from build123d import *

# Parameters (mm, degrees)
SKETCH_1_R               = 38.15
EXTRUDE_1_DEPTH          = 3
SKETCH_2_R               = 35.35
EXTRUDE_2_DEPTH          = 2
SKETCH_6_R               = 5.5
CUT_EXTRUDE_2_DEPTH      = 6
SKETCH_7_R               = 32.5
SKETCH_7_R_2             = 13.5
CUT_EXTRUDE_3_DEPTH      = 1
CUT_EXTRUDE_3_DEPTH_BACK = 6
EXTRUDE_4_DEPTH          = 5
PATTERN_CIRCULAR_3_COUNT = 6
MIRROR_1_COPY_1_DEPTH    = 5
MIRROR_1_COPY_2_DEPTH    = 5
MIRROR_1_COPY_3_DEPTH    = 5
MIRROR_1_COPY_4_DEPTH    = 5
MIRROR_1_COPY_5_DEPTH    = 5
SKETCH_9_R               = 1.6
CUT_EXTRUDE_4_DEPTH      = 6
FILLET_3_R               = 1.6
FILLET_4_R               = 1.6
SKETCH_11_R              = 12.05
CUT_EXTRUDE_6_DEPTH      = 2


with BuildPart() as part:
    # ｽｹｯﾁ1 → ﾎﾞｽ - 押し出し1 (new body)
    with BuildSketch(Plane.XY):
        Circle(SKETCH_1_R)
    extrude(amount=EXTRUDE_1_DEPTH)

    # ｽｹｯﾁ2 → ﾎﾞｽ - 押し出し2 (add)
    with BuildSketch(Plane.XY.offset(3)):
        Circle(SKETCH_2_R)
    extrude(amount=EXTRUDE_2_DEPTH)

    # ｽｹｯﾁ6 → ｶｯﾄ - 押し出し2 (cut, through all)
    with BuildSketch(Plane.XY.offset(5)):
        Circle(SKETCH_6_R)
    extrude(amount=-CUT_EXTRUDE_2_DEPTH, mode=Mode.SUBTRACT)

    # ｽｹｯﾁ7 → ｶｯﾄ - 押し出し3 (cut, two sides)
    with BuildSketch(Plane.XY.offset(5)) as cut_extrude_3_sk:
        Circle(SKETCH_7_R)
        Circle(SKETCH_7_R_2, mode=Mode.SUBTRACT)
    extrude(amount=CUT_EXTRUDE_3_DEPTH, mode=Mode.SUBTRACT)
    extrude(cut_extrude_3_sk.sketch, amount=-CUT_EXTRUDE_3_DEPTH_BACK, mode=Mode.SUBTRACT)

    # ｽｹｯﾁ8 → ﾎﾞｽ - 押し出し4 (add)
    with BuildSketch(Plane.XY.offset(5)):
        with BuildLine():
            Line((-12.910378376, 3.946153846), (-4.268742546, 32.218439395))
            ThreePointArc((-4.268742546, 32.218439395), (-2.139009075, 32.429533456), (0, 32.5))
            Line((0, 32.5), (-6.281364189, 11.949663758))
            ThreePointArc((-6.281364189, 11.949663758), (-10.396864354, 8.611342032), (-12.910378376, 3.946153846))
        make_face()
    extrude_4 = extrude(amount=-EXTRUDE_4_DEPTH)

    # 円形ﾊﾟﾀｰﾝ3: ﾎﾞｽ - 押し出し4 ×6 about axis
    pattern_circular_3_axis = Axis((0, 0, 0), (0, 0, 1))
    for i in range(1, PATTERN_CIRCULAR_3_COUNT):
        add(extrude_4.rotate(pattern_circular_3_axis, i * 360 / PATTERN_CIRCULAR_3_COUNT))

    # ﾐﾗｰ1: ﾎﾞｽ - 押し出し4 across plane
    add(extrude_4.mirror(Plane(origin=(0, 0, 0), x_dir=(0, 0, 1), z_dir=(1, 0, 0))))

    # ﾐﾗｰ1 copy 1 sketch → ﾐﾗｰ1 copy 1 (add)
    with BuildSketch(Plane(origin=(0, 0, 5), x_dir=(-0.5, 0.866025404, 0), z_dir=(0, 0, 1))):
        with BuildLine():
            Line((-12.910378376, -3.946153846), (-4.268742546, -32.218439395))
            ThreePointArc((-4.268742546, -32.218439395), (-2.139009075, -32.429533456), (0, -32.5))
            Line((0, -32.5), (-6.281364189, -11.949663758))
            ThreePointArc((-6.281364189, -11.949663758), (-10.396864354, -8.611342032), (-12.910378376, -3.946153846))
        make_face()
    extrude(amount=-MIRROR_1_COPY_1_DEPTH)

    # ﾐﾗｰ1 copy 2 sketch → ﾐﾗｰ1 copy 2 (add)
    with BuildSketch(Plane(origin=(0, 0, 5), x_dir=(0.5, 0.866025404, 0), z_dir=(0, 0, 1))):
        with BuildLine():
            Line((-12.910378376, -3.946153846), (-4.268742546, -32.218439395))
            ThreePointArc((-4.268742546, -32.218439395), (-2.139009075, -32.429533456), (0, -32.5))
            Line((0, -32.5), (-6.281364189, -11.949663758))
            ThreePointArc((-6.281364189, -11.949663758), (-10.396864354, -8.611342032), (-12.910378376, -3.946153846))
        make_face()
    extrude(amount=-MIRROR_1_COPY_2_DEPTH)

    # ﾐﾗｰ1 copy 3 sketch → ﾐﾗｰ1 copy 3 (add)
    with BuildSketch(Plane.XY.offset(5)):
        with BuildLine():
            Line((-12.910378376, -3.946153846), (-4.268742546, -32.218439395))
            ThreePointArc((-4.268742546, -32.218439395), (-2.139009075, -32.429533456), (0, -32.5))
            Line((0, -32.5), (-6.281364189, -11.949663758))
            ThreePointArc((-6.281364189, -11.949663758), (-10.396864354, -8.611342032), (-12.910378376, -3.946153846))
        make_face()
    extrude(amount=-MIRROR_1_COPY_3_DEPTH)

    # ﾐﾗｰ1 copy 4 sketch → ﾐﾗｰ1 copy 4 (add)
    with BuildSketch(Plane(origin=(0, 0, 5), x_dir=(0.5, -0.866025404, 0), z_dir=(0, 0, 1))):
        with BuildLine():
            Line((-12.910378376, -3.946153846), (-4.268742546, -32.218439395))
            ThreePointArc((-4.268742546, -32.218439395), (-2.139009075, -32.429533456), (0, -32.5))
            Line((0, -32.5), (-6.281364189, -11.949663758))
            ThreePointArc((-6.281364189, -11.949663758), (-10.396864354, -8.611342032), (-12.910378376, -3.946153846))
        make_face()
    extrude(amount=-MIRROR_1_COPY_4_DEPTH)

    # ﾐﾗｰ1 copy 5 sketch → ﾐﾗｰ1 copy 5 (add)
    with BuildSketch(Plane(origin=(0, 0, 5), x_dir=(-0.5, -0.866025404, 0), z_dir=(0, 0, 1))):
        with BuildLine():
            Line((-12.910378376, -3.946153846), (-4.268742546, -32.218439395))
            ThreePointArc((-4.268742546, -32.218439395), (-2.139009075, -32.429533456), (0, -32.5))
            Line((0, -32.5), (-6.281364189, -11.949663758))
            ThreePointArc((-6.281364189, -11.949663758), (-10.396864354, -8.611342032), (-12.910378376, -3.946153846))
        make_face()
    extrude(amount=-MIRROR_1_COPY_5_DEPTH)

    # ｽｹｯﾁ9 → ｶｯﾄ - 押し出し4 (cut, through all)
    with BuildSketch(Plane.XY.offset(5)):
        with Locations((-8.5, 0)):
            Circle(SKETCH_9_R)
        with Locations((0, 8.5)):
            Circle(SKETCH_9_R)
        with Locations((8.5, 0)):
            Circle(SKETCH_9_R)
        with Locations((0, -8.5)):
            Circle(SKETCH_9_R)
    extrude(amount=-CUT_EXTRUDE_4_DEPTH, mode=Mode.SUBTRACT)

    # ﾌｨﾚｯﾄ3
    fillet_3_edges = [part.edges().sort_by_distance(p)[0] for p in [
        (11.999058751, 6.9276598, 2.5),
        (9.230036516, 15.986892202, 2.5),
        (4.268742546, 32.218439395, 2.5),
        (15.725247398, -2.932347892, 2.5),
        (15.725247398, 2.932347892, 2.5),
        (18.460073032, 0, 2.5),
        (11.999058751, -6.9276598, 2.5),
        (30.03635826, 12.41238021, 2.5),
        (10.402111466, -12.152289781, 2.5),
        (9.230036516, -15.986892202, 2.5),
        (25.767615714, -19.806059185, 2.5),
        (-5.323135932, 15.084637673, 2.5),
        (-9.230036516, 15.986892202, 2.5),
        (0, 13.8553196, 2.5),
        (-25.767615714, 19.806059185, 2.5),
        (4.268742546, -32.218439395, 2.5),
        (30.03635826, -12.41238021, 2.5),
        (28.145825623, -16.25, 2.5),
        (25.767615714, 19.806059185, 2.5),
        (28.145825623, 16.25, 2.5),
        (-4.268742546, 32.218439395, 2.5),
        (0, 32.5, 2.5),
        (10.402111466, 12.152289781, 2.5),
        (5.323135932, 15.084637673, 2.5),
    ]]
    fillet(fillet_3_edges, radius=FILLET_3_R)

    # ﾌｨﾚｯﾄ4
    fillet_4_edges = [part.edges().sort_by_distance(p)[0] for p in [
        (5.323135932, -15.084637673, 2.5),
        (0, -13.8553196, 2.5),
        (-10.402111466, -12.152289781, 2.5),
        (-5.323135932, -15.084637673, 2.5),
        (-9.230036516, -15.986892202, 2.5),
        (-11.999058751, -6.9276598, 2.5),
        (-4.268742546, -32.218439395, 2.5),
        (-15.725247398, 2.932347892, 2.5),
        (-15.725247398, -2.932347892, 2.5),
        (-18.460073032, 0, 2.5),
        (-11.999058751, 6.9276598, 2.5),
        (-30.03635826, -12.41238021, 2.5),
        (-30.03635826, 12.41238021, 2.5),
        (-28.145825623, 16.25, 2.5),
        (-10.402111466, 12.152289781, 2.5),
        (-25.767615714, -19.806059185, 2.5),
        (-28.145825623, -16.25, 2.5),
        (0, -32.5, 2.5),
    ]]
    fillet(fillet_4_edges, radius=FILLET_4_R)

    # ｽｹｯﾁ11 → ｶｯﾄ - 押し出し6 (cut)
    with BuildSketch(Plane.XY.offset(5)):
        Circle(SKETCH_11_R)
    extrude(amount=-CUT_EXTRUDE_6_DEPTH, mode=Mode.SUBTRACT)


solid = part.part
The model under review builds one solid part; all positions refer to its coordinate system, in mm. A direction names the side the tool comes from. Round coordinates to 2 decimals unless told otherwise and drop trailing zeros. Write each loop counter-clockwise with the first axis right and the second up, starting at its lowest first coordinate (ties: lowest second). Pieces come first, ordered by that corner, then holes. Notation, with made-up numbers: M 22,-28.75 L 50,-28.75 A26 ccw 50,-4.75 Z; hole C 49.5,23 d3. An arc over 180 degrees is marked long. Use a Markdown table: item, result. Add a question column.
Q1. We need section B-B, the plane y = -25. State the section outline as (x, z) points, plus the area to 3 significant figures.
Q2. Machinability: for faces 1 (the face through (32.5, -0.1, 2.5)), 2 (the face through (-8.881, 8.144, 4.014)), which of the approach directions +Z, -Z, +X, -X, +Y, -Y give a long, thin tool a straight path to every point of the face, cutting with its end or side? Answer none if there is none.
Q3. The part is to be moulded in two halves that separate along Y. For faces 3 (the face through (24.39, -20.28, 2.46)), 4 (the face through (33.718, 10.618, 3.986)), 5 (the face through (15.74, -3.68, 2.46)), 6 (the face through (9, 14, 5)), say which applies: pulls with the +Y half, pulls with the -Y half, needs draft (parallel to the pull), parting line crosses it, or undercut.
Q4. Insertion check: pin 1 (1 mm diameter, centred on x = 10.5, z = 2, fed in from +Y); pin 2 (1 mm diameter, centred on y = -25, z = 4, fed in from +X); pin 3 (1 mm diameter, centred on x = -14.5, y = 16, fed in from -Z); pin 4 (3 mm diameter, centred on x = 8.5, y = 0, fed in from -Z). Each pin has a flat end and moves straight along its axis. Give the tip position at first contact, or say it passes through.
Q5. We need section A-A, the plane y = 0. Count the separate pieces of the cut face and the enclosed holes in it, plus the area to 3 significant figures.
Q6. To check wall thickness, follow line 1 (X direction, y = -29, z = 3.45); line 2 (X direction, y = 3.5, z = 1.3); line 3 (X direction, y = 24, z = 3.2). State the ranges of each line that lie inside material, in increasing order.
Findings below:
| question | item | result |
|---|---|---|
| 1 | outline | M -28.82,0 L -20.77,0 L -20.77,5 L -24.99,5 L -24.99,3 L -28.82,3 Z; M -6.48,0 L -2.29,0 L -2.29,5 L -6.48,5 Z; M 2.29,0 L 6.48,0 L 6.48,5 L 2.29,5 Z; M 20.77,0 L 28.82,0 L 28.82,3 L 24.99,3 L 24.99,5 L 20.77,5 Z |
| 1 | area | 107 mm² |
| 2 | face 1 | +Z, -Z |
| 2 | face 2 | +Z |
| 3 | face 3 | undercut |
| 3 | face 4 | parting line crosses it |
| 3 | face 5 | undercut |
| 3 | face 6 | needs draft |
| 4 | pin 1 | stops at y = 36.82 |
| 4 | pin 2 | stops at x = 25.48 |
| 4 | pin 3 | stops at z = 0 |
| 4 | pin 4 | passes through |
| 5 | separate pieces | 6 |
| 5 | enclosed holes | 0 |
| 5 | area | 135 mm² |
| 6 | line 1 | x = -20.21 to -14.67, -5.25 to 5.25, 14.67 to 20.21 |
| 6 | line 2 | x = -37.99 to -32.31, -21.72 to -4.24, 4.24 to 21.72, 32.31 to 37.99 |
| 6 | line 3 | x = -25.95 to -21.91, -6.78 to -2.6, 2.6 to 6.78, 21.91 to 25.95 |
